Geometry: final body of the model. Coordinates: model frame, mm. Face numbers are marked on the shaded views. Coordinates: 2 decimals unless noted, no trailing zeros. Order: outer loops, then holes, each group sorted by start corner. A loop starts at its lowest first (then second) coordinate and runs counter-clockwise, first axis right, second up. Notation, with made-up numbers: M 10.5,-33 L 56.5,-33 A10 ccw 56.5,-26 Z; hole C 58,18.25 d11. An arc over 180 degrees is marked long. Use CSV: the item, a comma, the result in double quotes. Start each with the question number.
Q1. Section query B-B, the plane x = -381. Output: boundary loops of the cut face in (y, z), and give its area (3 significant figures).
Q2. Section query D-D, the plane z = -19. Output: boundary loops of the cut face in (x, y).
Q3. Ray query, probe 1 along X at (y, z) = (132, -110.25); probe 2 along Z at (x, y) = (208, 92); probe 3 along Z at (x, y) = (-40.5, -18). Return the intervals inside material, ascending.
Q4. First-contact query: P1, Ø12, axis at x = 30, y = -25.5, coming from the +Z side; P2, Ø5, axis at x = 29, z = 32.5, coming from the +Y side; P3, Ø7, axis at x = 270, y = 132, coming from the -Z side; P4, Ø6, axis at x = -159, z = -62.5, coming from the -Y side. Flat tips, straight axial feed; report the tip coordinate or a pass-through.
Q5. Mould query, pull axis Z, two halves, no side actions, for the marked faces 1, 2, 3 and 4. Classes: +Z half, -Z half, draft (parallel to the pull), parting line (faces both ways), or undercut.
Q6. Section query C-C, the plane y = -87.5. Output: boundary loops of the cut face in (x, z).
Q7. Section query A-A, the plane y = 115.5. Output: boundary loops of the cut face in (x, z), and give its area (3 significant figures).
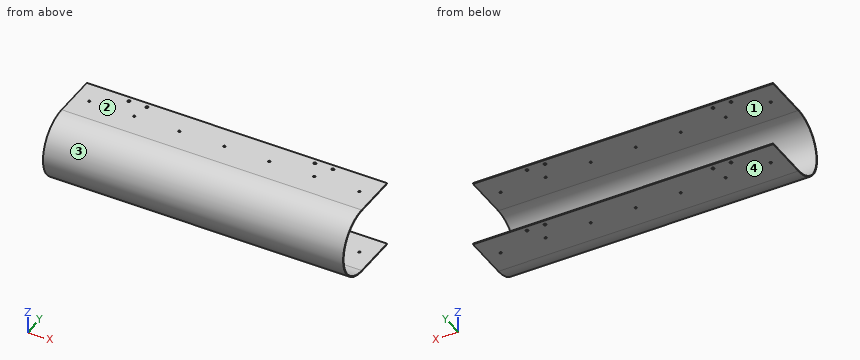
from build123d import *

# Parameters (mm, degrees)
OTHER_START              = -500
OTHER_2_DEPTH            = 1000
CUT_EXTRUDE_4_DEPTH      = 534.686237409
CUT_EXTRUDE_4_DEPTH_BACK = 534.686237409
SKETCH_13_R              = 3.5
SKETCH_13_R_2            = 4.5


# Read off the part's stored shape, not the designer's step: Элемент по сечениям сгиба2
with BuildPart() as part:
    # Other 2 outline → Other 2 (new body)
    with BuildSketch(Plane.YZ.offset(OTHER_START)):
        with BuildLine():
            Line((0, -111), (150, -111))
            Line((150, -111), (150, -108))
            Line((150, -108), (0, -108))
            ThreePointArc((0, -108), (-108, 0), (0, 108))
            Line((0, 108), (150, 108))
            Line((150, 108), (150, 111))
            Line((150, 111), (0, 111))
            ThreePointArc((0, 111), (-111, 0), (0, -111))
        make_face()
    extrude(amount=OTHER_2_DEPTH)

    # Эскиз13 → Вырез-Вытянуть4 (cut, two sides: drawn at the far end of the back side and taken through both)
    with BuildSketch(Plane.XY.offset(-CUT_EXTRUDE_4_DEPTH_BACK)):
        with Locations((450, 75)):
            Circle(SKETCH_13_R)
        with Locations((300, 75)):
            Circle(SKETCH_13_R)
        with Locations((150, 75)):
            Circle(SKETCH_13_R)
        with Locations((0, 75)):
            Circle(SKETCH_13_R)
        with Locations((-150, 75)):
            Circle(SKETCH_13_R)
        with Locations((-300, 75)):
            Circle(SKETCH_13_R)
        with Locations((-450, 75)):
            Circle(SKETCH_13_R)
        with Locations((330, 132)):
            Circle(SKETCH_13_R_2)
        with Locations((270, 132)):
            Circle(SKETCH_13_R_2)
        with Locations((-350, 132)):
            Circle(SKETCH_13_R_2)
        with Locations((-290, 132)):
            Circle(SKETCH_13_R_2)
    extrude(amount=CUT_EXTRUDE_4_DEPTH + CUT_EXTRUDE_4_DEPTH_BACK, mode=Mode.SUBTRACT)


solid = part.part
Responses:
1,outline,"M 0,-111 L 150,-111 L 150,-108 L 0,-108 A108 cw 0,108 L 150,108 L 150,111 L 0,111 A111 ccw Z"
1,area,"1,930 mm²"
2,outline,"M -500,-109.36 L 500,-109.36 L 500,-106.32 L -500,-106.32 Z"
3,probe 1,"x = -500 to -354.5, -345.5 to -294.5, -285.5 to 265.5, 274.5 to 325.5, 334.5 to 500"
3,probe 2,"z = -111 to -108, 108 to 111"
3,probe 3,"z = -109.53 to -106.49, 106.49 to 109.53"
4,P1,"stops at z = 109.27"
4,P2,"stops at y = -102.17"
4,P3,"passes through"
4,P4,"stops at y = -93.71"
5,face 1,"undercut"
5,face 2,"+Z half"
5,face 3,"parting line"
5,face 4,"-Z half"
6,outline,"M -500,-68.3 L 500,-68.3 L 500,-63.31 L -500,-63.31 Z; M -500,63.31 L 500,63.31 L 500,68.3 L -500,68.3 Z"
7,outline,"M -500,-111 L 500,-111 L 500,-108 L -500,-108 Z; M -500,108 L 500,108 L 500,111 L -500,111 Z"
7,area,"6,000 mm²"
